Here's the drawing with two shaded views (mm, measured from the low corner). I have some questions. A direction names the side the tool comes from. Coordinates: 2 decimals unless noted, no trailing zeros. Write each loop counter-clockwise with the first axis right and the second up, starting at its lowest first coordinate (ties: lowest second). Pieces come first, ordered by that corner, then holes.
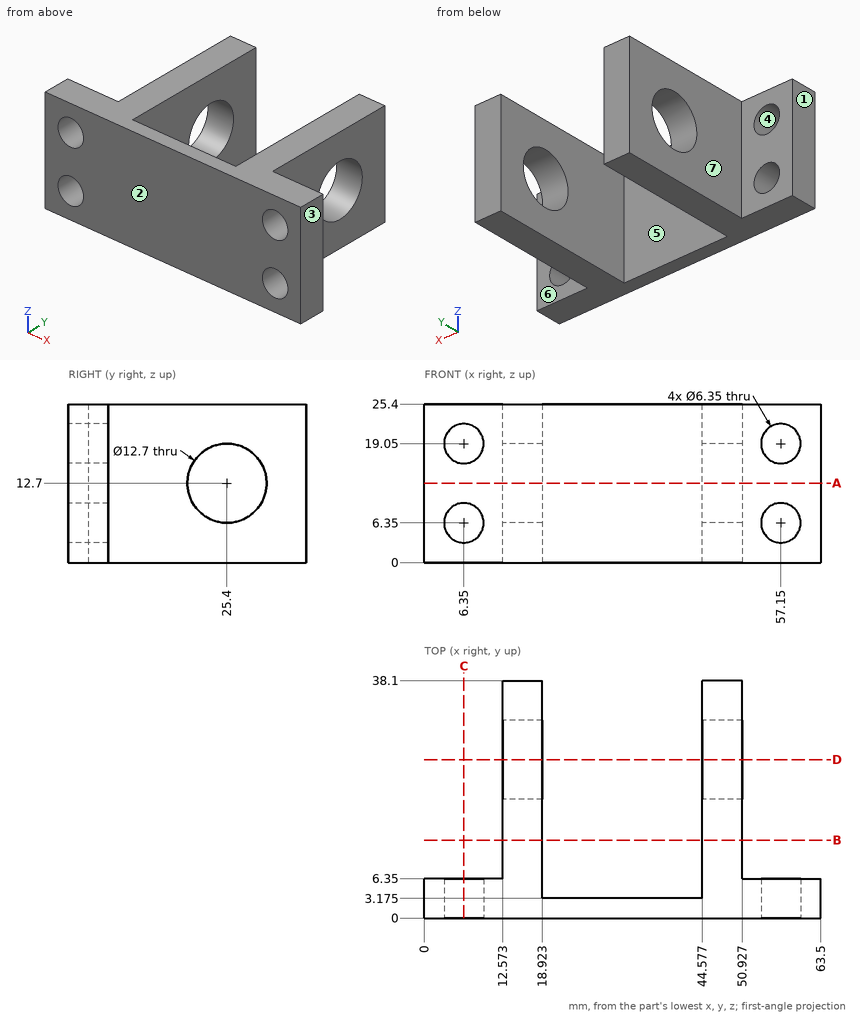
Item 1: I want a section at A-A, the plane z = 12.7. List the corners of the cut face in (x, y) for me (3 decimals).
Item 2: I want a section at D-D, the plane y = 25.4. List the corners of the cut face in (x, z) for me, then the cut area to 3 significant figures.
Item 3: Will these pins go through, and if not, where does the flat tip stop? pin 1 Ø1 at (y, z) = (17.5, 3.5) entering from -X; pin 2 Ø12 at (y, z) = (13.5, 12) entering from +X; pin 3 Ø5.5 at (x, z) = (6.35, 6.35) entering from -Y; pin 4 Ø7.5 at (x, z) = (29, 12.5) entering from +Y (3 decimals).
Item 4: I want a section at B-B, the plane y = 12.5. List the corners of the cut face in (x, z) for me.
Item 5: I want a section at C-C, the plane x = 6.35. List the corners of the cut face in (y, z) for me (3 decimals).
Item 6: Which directions (+Z, -Z, +X, -X, +Y, -Y) give clear straight access to the entire face, cutting with the end or side of a thin tool? Please do the marked faces 5, 6 and 7.
Item 7: If I drill on line 1 along X through (y, z) = (3.25, 6.35) (3 decimals); line 2 along Z through (x, y) = (57, 5); line 3 along X through (y, z) = (17, 23.75), over which ranges is the centre line in solid material (lowest first)?
Item 8: If we mould it in two halves opening along X, with no side actions, what happens to the marked faces 1, 2, 3 and 4? For each: released by +X, released by -X, zero draft, split by the parting line, or undercut.
Taken from the geometry:
1. outline: (0, 0) - (63.5, 0) - (63.5, 6.35) - (50.927, 6.35) - (50.927, 19.05) - (44.577, 19.05) - (44.577, 3.175) - (18.923, 3.175) - (18.923, 19.05) - (12.573, 19.05) - (12.573, 6.35) - (0, 6.35) - close; (12.573, 31.75) - (18.923, 31.75) - (18.923, 38.1) - (12.573, 38.1) - close; (44.577, 31.75) - (50.927, 31.75) - (50.927, 38.1) - (44.577, 38.1) - close
2. outline: (12.57, 0) - (18.92, 0) - (18.92, 6.35) - (12.57, 6.35) - close; (12.57, 19.05) - (18.92, 19.05) - (18.92, 25.4) - (12.57, 25.4) - close; (44.58, 0) - (50.93, 0) - (50.93, 6.35) - (44.58, 6.35) - close; (44.58, 19.05) - (50.93, 19.05) - (50.93, 25.4) - (44.58, 25.4) - close
2. area: 161 mm2
3. pin 1: stops at x = 12.57
3. pin 2: stops at x = 50.93
3. pin 3: passes through
3. pin 4: stops at y = 3.175
4. outline: (12.57, 0) - (18.92, 0) - (18.92, 25.4) - (12.57, 25.4) - close; (44.58, 0) - (50.93, 0) - (50.93, 25.4) - (44.58, 25.4) - close
5. outline: (0, 0) - (6.35, 0) - (6.35, 3.175) - (0, 3.175) - close; (0, 9.525) - (6.35, 9.525) - (6.35, 15.875) - (0, 15.875) - close; (0, 22.225) - (6.35, 22.225) - (6.35, 25.4) - (0, 25.4) - close
6. face 5: +Z, -Z, +Y
6. face 6: +Z, -Z, +X, +Y
6. face 7: +Z, -Z, -X, +Y
7. line 1: x = 0 to 3.175, 9.525 to 18.923, 44.577 to 53.975, 60.325 to 63.5
7. line 2: z = 0 to 3.18, 9.52 to 15.88, 22.22 to 25.4
7. line 3: x = 12.57 to 18.92, 44.58 to 50.93
8. face 1: released by -X
8. face 2: zero draft
8. face 3: released by +X
8. face 4: undercut
